Geometry check sheet. Reference: the model listing, model coordinates, mm. Face numbers are marked on the shaded views. A direction names the side the tool comes from. Give positions to 0.01 mm unless a question says otherwise; leave off trailing zeros. Write each loop counter-clockwise with the first axis right and the second up, starting at its lowest first coordinate (ties: lowest second). Pieces come first, ordered by that corner, then holes. Notation, with made-up numbers: M 27.5,-33 L 71.5,-33 A20 ccw 71.5,-15 Z; hole C -33.5,28.25 d10. An arc over 180 degrees is marked long. Write each question's results on one line, items separated by ' | '.
```python
from build123d import *

# Parameters (mm, degrees)
SKETCH1_W           = 72
SKETCH1_H           = 40
BOSS_EXTRUDE2_DEPTH = 40
SKETCH3_R           = 9
CUT_EXTRUDE2_DEPTH  = 4
SKETCH7_W           = 72
SKETCH7_H           = 40
BOSS_EXTRUDE5_DEPTH = 1


with BuildPart() as part:
    # Sketch1 → Boss-Extrude2 (new body)
    with BuildSketch(Plane.XY):
        with BuildLine():
            Line((-34.5, -22.5), (34.5, -22.5))
            ThreePointArc((34.5, -22.5), (36.621320344, -21.621320344), (37.5, -19.5))
            Line((37.5, -19.5), (37.5, 19.5))
            ThreePointArc((37.5, 19.5), (36.621320344, 21.621320344), (34.5, 22.5))
            Line((34.5, 22.5), (-34.5, 22.5))
            ThreePointArc((-34.5, 22.5), (-36.621320344, 21.621320344), (-37.5, 19.5))
            Line((-37.5, 19.5), (-37.5, -19.5))
            ThreePointArc((-37.5, -19.5), (-36.621320344, -21.621320344), (-34.5, -22.5))
        make_face()
        Rectangle(SKETCH1_W, SKETCH1_H, mode=Mode.SUBTRACT)
    extrude(amount=BOSS_EXTRUDE2_DEPTH)

    # Sketch3 → Cut-Extrude2 (cut)
    with BuildSketch(Plane(origin=(0, -20, 0), x_dir=(1, 0, 0), z_dir=(0, 1, 0))):
        with Locations(Location((-0.42510875, -20, 0), (0, 0, 270))):
            Circle(SKETCH3_R)
    extrude(amount=-CUT_EXTRUDE2_DEPTH, mode=Mode.SUBTRACT)

    # Sketch7 → Boss-Extrude5 (add)
    with BuildSketch(Plane.XY):
        Rectangle(SKETCH7_W, SKETCH7_H)
    extrude(amount=BOSS_EXTRUDE5_DEPTH)


solid = part.part
```
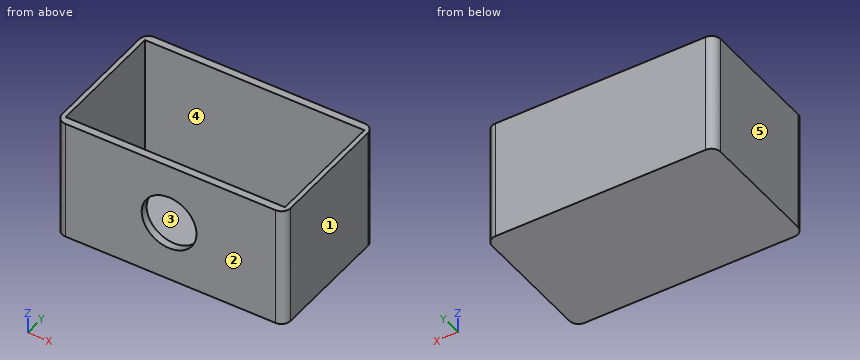
Q1. Section check D-D (y = 4). Enter the section's corners in (x, z).
Answer key:
outline: M -37.5,0 L 37.5,0 L 37.5,40 L 36,40 L 36,1 L -36,1 L -36,40 L -37.5,40 Z
Q2. Release check for a two-part mould opening along Y. For the marked faces 1, 2 and 3 record: released by +Y, released by -Y, zero draft, split by the parting line, or undercut.
Answer key:
face 1: zero draft | face 2: released by -Y | face 3: undercut
Q3. Section check C-C (z = 20). Enter the section's corners in (x, y).
Answer key:
outline: M -37.5,-19.5 A3 ccw -34.5,-22.5 L -9.43,-22.5 L -9.43,-20 L -36,-20 L -36,20 L 36,20 L 36,-20 L 8.57,-20 L 8.57,-22.5 L 34.5,-22.5 A3 ccw 37.5,-19.5 L 37.5,19.5 A3 ccw 34.5,22.5 L -34.5,22.5 A3 ccw -37.5,19.5 Z
Q4. Material ranges on probe 1 along X at (y, z) = (-12.5, 32.5); probe 2 along Y at (x, z) = (17.5, 7); probe 3 along Z at (x, y) = (-29, 5.5), recorded low to high. Write a range as [from, to].
Answer key:
probe 1: x = [-37.5, -36], [36, 37.5] | probe 2: y = [-22.5, -20], [20, 22.5] | probe 3: z = [0, 1]
Q5. Section check B-B (x = 25). Enter the section's corners in (y, z).
Answer key:
outline: M -22.5,0 L 22.5,0 L 22.5,40 L 20,40 L 20,1 L -20,1 L -20,40 L -22.5,40 Z
Q6. Section check A-A (z = 5.5). Enter the section's corners in (x, y), then the cut area to 3 significant figures.
Answer key:
outline: M -37.5,-19.5 A3 ccw -34.5,-22.5 L 34.5,-22.5 A3 ccw 37.5,-19.5 L 37.5,19.5 A3 ccw 34.5,22.5 L -34.5,22.5 A3 ccw -37.5,19.5 Z; hole M -36,-20 L 36,-20 L 36,20 L -36,20 Z | area: 487 mm2
Q7. Depth check by flat-ended pin: P1, Ø20, axis at x = 16, y = -3, coming from the +Z side. Enter the tip coordinate at first touch or a pass-through.
Answer key:
P1: stops at z = 1
Q8. Access from +Z, -Z, +X, -X, +Y, -Y to the whole of each face (thin tool, end or side, straight path). Record for the marked faces 4 and 5.
Answer key:
face 4: +Z | face 5: +Z, -Z, -X, +Y, -Y
